Verification items for this drawing (mm, ordinates from the low corner). Coordinates: 2 decimals unless noted, no trailing zeros. Order: outer loops, then holes, each group sorted by start corner. A loop starts at its lowest first (then second) coordinate and runs counter-clockwise, first axis right, second up. Notation, with made-up numbers: M 17,28 L 22,28 A18 ccw 22,54 Z; hole C 84,-1.5 d11. An arc over 180 degrees is marked long. One line per item, written item: value. Start each with the question number.
1) Sectioned sample at C-C, the plane x = 46. Enter the section's corners in (y, z) (1 decimal).
2) Thickness scan on L1, parallel to Z at x = 40, y = 1.55 (1 decimal); L2, parallel to X at y = 1.3, z = 19; L3, parallel to Z at x = 76.5, y = 0.6. Record the ranges inside material, lowest first. Write a range as from..to.
3) Go/stop test with a flat-tipped pin: P1, Ø1.8, axis at x = 46, z = 46.275, coming from the -Y side. Record where the tip stops, or that it passes through.
4) Sectioned sample at A-A, the plane x = 30. Enter the section's corners in (y, z).
5) Sectioned sample at D-D, the plane y = 0.5. State how many separate pieces and enclosed holes the cut face has, then the cut area to 3 significant figures.
6) Sectioned sample at B-B, the plane z = 10. Enter the section's corners in (x, y).
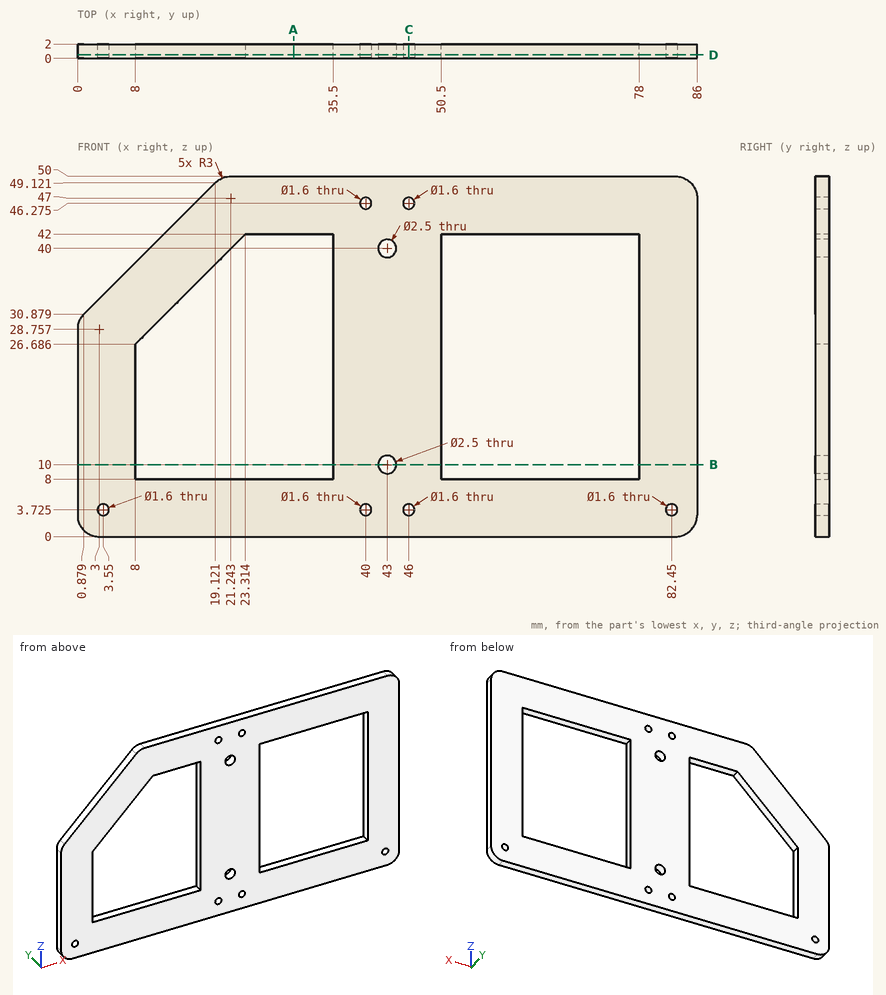
Final values:
1. outline: M 0,0 L 2,0 L 2,2.9 L 0,2.9 Z; M 0,4.5 L 2,4.5 L 2,45.5 L 0,45.5 Z; M 0,47.1 L 2,47.1 L 2,50 L 0,50 Z
2. L1: z = 0..2.9, 4.5..45.5, 47.1..50
2. L2: x = 0..8, 35.5..50.5, 78..86
2. L3: z = 0..8, 42..50
3. P1: stops at y = 0
4. outline: M 0,0 L 2,0 L 2,8 L 0,8 Z; M 0,42 L 2,42 L 2,50 L 0,50 Z
5. separate pieces: 1
5. enclosed holes: 10
5. area: 2,320 mm^2
6. outline: M 0,0 L 8,0 L 8,2 L 0,2 Z; M 35.5,0 L 41.75,0 L 41.75,2 L 35.5,2 Z; M 44.25,0 L 50.5,0 L 50.5,2 L 44.25,2 Z; M 78,0 L 86,0 L 86,2 L 78,2 Z
